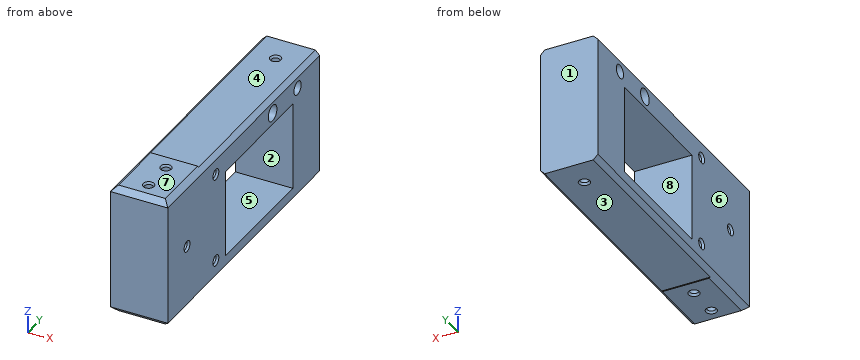
Solid Edge part; units mm, degrees
sketch "Sketch1" plane through (0, 0, 0) normal (0, 0, 1) x (1, 0, 0)
  line L0 (-16, -30) -> (16, -30)
  line L1 (16, -30) -> (16, 30)
  line L2 (16, 30) -> (-16, 30)
  line L3 (-16, 30) -> (-16, -30)
  dimension "D1" = 16
  dimension "D2" = 16
extrude "Protrusion1" add sketch "Sketch1" along normal blind 73
sketch "Sketch2" plane through (0, 0, 73) normal (0, 0, 1) x (1, 0, 0)
  circle A0 centre (0, -20) radius 2.35
  circle A1 centre (0, -2) radius 2.35
extrude "Cutout1" cut sketch "Sketch2" against normal through all
chamfer "Fase_3" distance 0.7 angle 60 4 edges at (-2.35, -2, 73) (-2.35, -20, 73) (-2.35, -20, 0) (-2.35, -2, 0) measured on face at (-10.9867, -19.4, 73) measured on face at (-10.9867, -19.4, 0)
chamfer "Fase_6" distance 3 angle 45 4 edges at (-16, 0, 73) (-16, 0, 0) (16, 0, 73) (16, 0, 0)
chamfer "Fase_7" distance 3 angle 45 2 edges at (0, -30, 73) (0, -30, 0)
sketch "Sketch3" plane through (-16, 0, 36.5) normal (-1, 0, 0) x (0, -1, 0)
  circle A0 centre (-20, 25) radius 2.35
  circle A1 centre (-20, -25) radius 2.35
  circle A2 centre (10, 0) radius 2.35
  dimension "D1" = 20
extrude "Cutout2" cut sketch "Sketch3" against normal through all
chamfer "Fase_9" distance 0.7 angle 60 6 edges at (-16, 22.35, 61.5) (-16, -7.65, 36.5) (-16, 22.35, 11.5) (16, 20, 59.15) (16, 20, 9.15) (16, -10, 34.15) measured on face at (-16, 20.6, 58.1633) measured on face at (16, -20.6, 58.1633)
sketch "Sketch4" plane through (-16, 0, 36.5) normal (-1, 0, 0) x (0, -1, 0)
  line L0 (-6.5, 36.5) -> (-30, 36.5)
  line L1 (-30, 36.5) -> (-30, 36)
  line L2 (-30, 36) -> (-6.5, 36)
  line L3 (-6.5, 36) -> (-6.5, 36.5)
  line L4 (-30, -36.5) -> (-6.5, -36.5)
  line L5 (-6.5, -36.5) -> (-6.5, -36)
  line L6 (-6.5, -36) -> (-30, -36)
  line L7 (-30, -36) -> (-30, -36.5)
  dimension "D1" = 30
  dimension "D2" = 30
extrude "Cutout3" cut sketch "Sketch4" against normal through all
sketch "Sketch5" plane through (0, 30, 36.5) normal (0, 1, 0) x (1, 0, 0)
  line L0 (-16, 33.5) -> (-13.5, 36)
  line L1 (-13.5, 36) -> (13.5, 36)
  line L2 (13.5, 36) -> (16, 33.5)
  line L3 (16, 33.5) -> (16, -33.5)
  line L4 (16, -33.5) -> (13.5, -36)
  line L5 (13.5, -36) -> (-13.5, -36)
  line L6 (-13.5, -36) -> (-16, -33.5)
  line L7 (-16, -33.5) -> (-16, 33.5)
extrude "Extrusionsausprägung_2" add sketch "Sketch5" along normal blind 26
sketch "Sketch6" plane through (0, 56, 36.5) normal (0, 1, 0) x (-1, 0, 0)
  line L0 (-13.5, 36) -> (-16, 33.5)
  line L1 (-16, 33.5) -> (-16, -33.5)
  line L2 (-16, -33.5) -> (-13.5, -36)
  line L3 (-13.5, -36) -> (13.5, -36)
  line L4 (13.5, -36) -> (16, -33.5)
  line L5 (16, -33.5) -> (16, 33.5)
  line L6 (16, 33.5) -> (13.5, 36)
  line L7 (13.5, 36) -> (-13.5, 36)
extrude "Extrusionsausprägung_3" add sketch "Sketch6" along normal blind 72
sketch "Sketch7" plane through (16, 47, 36.5) normal (1, 0, 0) x (0, 1, 0)
  line L0 (-17, 21) -> (53, 21)
  line L1 (53, 21) -> (53, -28)
  line L2 (53, -28) -> (-17, -28)
  line L3 (-17, -28) -> (-17, 21)
  dimension "D1" = 17
extrude "Cutout4" cut sketch "Sketch7" against normal through all
sketch "Sketch8" plane through (0, 65.25, 72.5) normal (0, 0, 1) x (0, 1, 0)
  circle A0 centre (46.75, 0) radius 2.35
  dimension "D1" = 46.75
extrude "Cutout5" cut sketch "Sketch8" against normal through all
chamfer "Fase_11" distance 0.7 angle 60 2 edges at (-2.35, 112, 0.5) (0, 109.65, 72.5) measured on face at (8.73, 108.965, 72.5) measured on face at (8.73, 25.535, 0.5)
sketch "Sketch9" plane through (-16, 49, 36.5) normal (-1, 0, 0) x (0, -1, 0)
  circle A0 centre (-56, 27.5) radius 3.75
extrude "Cutout6" cut sketch "Sketch9" against normal through all
sketch "Sketch10" plane through (-16, 49, 36.5) normal (-1, 0, 0) x (0, -1, 0)
  circle A0 centre (-30, 27.5) radius 4.5
extrude "Cutout7" cut sketch "Sketch10" against normal through all
properties material "Nylon, allgemein"
Verification items for the finished model (mm, model axes). Face numbers are marked on the shaded views. A direction names the side the tool comes from. Give positions to 0.01 mm unless a question says otherwise; leave off trailing zeros. Order: outer loops, then holes, each group sorted by start corner. A loop starts at its lowest first (then second) coordinate and runs counter-clockwise, first axis right, second up. Notation, with made-up numbers: M 84.5,-12 L 120.5,-12 A10 cw 120.5,-6 Z; hole C 18.5,32 d6. An arc over 180 degrees is marked long. Return JSON: item names as keys, results as strings. Group by question number.
1) Go/stop test with flat-tipped pins: pin 1 Ø4 at (x, y) = (0, -2) entering from +Z; pin 2 Ø6 at (x, y) = (0, -20) entering from -Z; pin 3 Ø8 at (x, y) = (-3, 57.5) entering from +Z; pin 4 Ø3 at (x, y) = (3, 41.5) entering from -Z. Record where each tip stops, or that it passes through.
2) Access from +Z, -Z, +X, -X, +Y, -Y to the whole of each face (thin tool, end or side, straight path). Record for the marked faces 1, 2, 3 and 4.
3) Section check B-B on y = 79. Record the cut outline in (x, z).
4) Section check D-D on y = -20. Record the cut outline in (x, z), and give its area (3 significant figures).
5) Scan lines: line 1 (Z direction, x = -2, y = 79); line 2 (Z direction, x = -0.5, y = 32.5); line 3 (Y direction, x = 13.5, z = 38). Record each from-to range of solid material in increasing order.
6) Section check C-C on x = -11. Record the cut outline in (y, z).
7) Section check A-A on z = 26.5. Record the cut outline in (x, y).
8) Mould release check, pull along Z, two halves, no side actions. Record for the marked faces 5, 6, 7 and 8: pulls with the +Z half, pulls with the -Z half, needs draft (parallel to the pull), parting line crosses it, or undercut.
Answer block:
{
 "1": {"pin 1": "passes through", "pin 2": "stops at z = 0.09", "pin 3": "stops at z = 72.5", "pin 4": "stops at z = 0.5"},
 "2": {"face 1": "+Z, -Z, +X, -X, +Y", "face 2": "+X, -X", "face 3": "-Z, +X, -X, +Y", "face 4": "+Z, +X, -X, +Y"},
 "3": {"outline": "M -16,3 L -13.5,0.5 L 13.5,0.5 L 16,3 L 16,8.5 L -16,8.5 Z; M -16,57.5 L 16,57.5 L 16,59.5 L -16,59.5 Z; M -16,68.5 L 16,68.5 L 16,70 L 13.5,72.5 L -13.5,72.5 L -16,70 Z"},
 "4": {"outline": "M -16,3 L -13,0 L -3.05,0 L -2.35,1.21 L -2.35,71.79 L -3.05,73 L -13,73 L -16,70 Z; M 2.35,1.21 L 3.05,0 L 13,0 L 16,3 L 16,70 L 13,73 L 3.05,73 L 2.35,71.79 Z", "area": "1,970 mm^2"},
 "5": {"line 1": "z = 0.5 to 8.5, 57.5 to 59.5, 68.5 to 72.5", "line 2": "z = 0.5 to 8.5, 57.5 to 72.5", "line 3": "y = -30 to -11.81, -8.19 to 30, 100 to 128"},
 "6": {"outline": "M -30,3 L -27,0 L 6.5,0 L 6.5,0.5 L 128,0.5 L 128,72.5 L 6.5,72.5 L 6.5,73 L -27,73 L -30,70 Z; hole C -10,36.5 d4.7; hole C 20,11.5 d4.7; hole C 20,61.5 d4.7; hole M 30,8.5 L 100,8.5 L 100,57.5 L 30,57.5 Z; hole C 79,64 d9; hole C 105,64 d7.5"},
 "7": {"outline": "M -16,-30 L 16,-30 L 16,30 L -16,30 Z; M -16,100 L 16,100 L 16,128 L -16,128 Z; hole C 0,-20 d4.7; hole C 0,-2 d4.7; hole C 0,112 d4.7"},
 "8": {"face 5": "undercut", "face 6": "needs draft", "face 7": "pulls with the +Z half", "face 8": "undercut"}
}
